Autodesk Inventor part; units mm, degrees
ref_plane "YZ Plane" through (0, 0, 0) normal (1, 0, 0) x (0, 1, 0)
ref_plane "XZ Plane" through (0, 0, 0) normal (0, 1, 0) x (-1, 0, 0)
ref_plane "XY Plane" through (0, 0, 0) normal (0, 0, 1) x (1, 0, 0)
sketch "Esboço4" plane through (0, 0, 0) normal (0, 0, 1) x (1, 0, 0)
  point P0 (0, 0)
  point P1 (43.221, 21.8373)
  point P2 (101.0161, 22.7479)
  point P3 (77.0161, 22.7479)
sketch "Esboço5" plane through (0, 0, 0) normal (0, 0, 1) x (1, 0, 0)
  line L0 (46.357, -8.7268) -> (46.357, 6.1732)
  line L1 (66.357, 6.1732) -> (66.357, -8.7268)
  line L2 (46.357, 6.1732) -> (44.357, 6.1732)
  line L3 (44.357, 6.1732) -> (44.357, -8.7268)
  line L4 (44.357, -8.7268) -> (46.357, -8.7268)
  line L5 (56.357, 6.1732) -> (56.357, -8.7268)
  circle A0 centre (42.407, -1.2768) radius 1.4
  line L6 (39.007, -1.2768) -> (44.357, -6.6268)
  line L7 (39.007, -1.2768) -> (46.573, -1.2768) construction
  line L8 (39.007, -1.2768) -> (39.007, 2.1232)
  line L9 (39.007, 2.1232) -> (44.357, 2.1232)
  line L10 (66.357, -8.7268) -> (66.357, 6.1732)
  line L11 (66.357, 6.1732) -> (68.357, 6.1732)
  line L12 (68.357, 6.1732) -> (68.357, -8.7268)
  line L13 (68.357, -8.7268) -> (66.357, -8.7268)
  circle A1 centre (70.307, -1.2768) radius 1.4
  line L14 (73.707, -1.2768) -> (68.357, -6.6268)
  line L15 (73.707, -1.2768) -> (66.1409, -1.2768) construction
  line L16 (73.707, -1.2768) -> (73.707, 2.1232)
  line L17 (73.707, 2.1232) -> (68.357, 2.1232)
  point P0 (0, 0)
  dimension "d23" = 20
  dimension "d29" = 2
  dimension "d35" = 45
extrude "Extrusão4" add sketch "Esboço5" along normal blind 2
sketch "Esboço6" plane through (0, 0, 2) normal (0, 0, 1) x (1, 0, 0)
  line L0 (46.357, 6.1732) -> (44.357, 6.1732)
  line L1 (46.357, 6.1732) -> (44.357, 6.1732)
  line L2 (44.357, -8.7268) -> (46.357, -8.7268)
  line L3 (46.357, -8.7268) -> (46.357, 6.1732)
  line L4 (44.357, 6.1732) -> (44.357, -8.7268)
  line L5 (46.357, -8.7268) -> (44.357, -8.7268)
  line L6 (66.357, 6.1732) -> (66.357, -8.7268)
  line L7 (68.357, 6.1732) -> (66.357, 6.1732)
  line L8 (66.357, 6.1732) -> (68.357, 6.1732)
  line L9 (68.357, 6.1732) -> (68.357, -8.7268)
  line L10 (68.357, -8.7268) -> (66.357, -8.7268)
  line L11 (66.357, -8.7268) -> (66.357, 6.1732)
  point P0 (0, 0)
extrude "Extrusão5" add sketch "Esboço6" along normal blind 11
sketch "Esboço7" plane through (0, 0, 13) normal (0, 0, 1) x (1, 0, 0)
  line L0 (44.357, 6.1732) -> (44.357, 2.1232)
  line L1 (68.357, -8.7268) -> (68.357, 6.1732)
  line L2 (44.357, 6.1732) -> (68.357, 6.1732)
  line L3 (68.357, 6.1732) -> (68.357, -8.7268)
  line L4 (68.357, -8.7268) -> (44.357, -8.7268)
  line L5 (44.357, -8.7268) -> (44.357, 6.1732)
  point P0 (0, 0)
extrude "Extrusão6" add sketch "Esboço7" along normal blind 2
chamfer "Chanfro1" distance 1 angle 45 1 edges at (68.907, -1.2768, 2)
chamfer "Chanfro2" distance 1 angle 45 1 edges at (41.007, -1.2768, 2)
properties part number "protetor_luz"
Input: part model. Units: mm. Frame: model coordinates. A direction names the side the tool comes from. Give positions to 0.01 mm unless a question says otherwise; leave off trailing zeros. Write each loop counter-clockwise with the first axis right and the second up, starting at its lowest first coordinate (ties: lowest second). Pieces come first, ordered by that corner, then holes. Notation, with made-up numbers: (-1, 7) -> (9, 7) arc R21 cw to (9, 35) -> close; hole circle Ø2 at (52.25, 74.25). An arc over 180 degrees is marked (long way). Use one line per item in the form item = value. Start each with the question number.
1) Pin query (flat end, axial travel): pin 1 (6 mm diameter, centred on y = -4.5, z = 2.5, fed in from -X); pin 2 (1.5 mm diameter, centred on y = -6.5, z = 7, fed in from -X); pin 3 (0.6 mm diameter, centred on x = 42.5, z = 1.5, fed in from +Y). Return the tip coordinate at first contact, or that it passes through.
2) Section query A-A on z = 9. Return the cut outline in (x, y).
3) Set-up query: faces 1 (the flat face through (42, 2.123, 1)), 2 (the flat face through (73, -1, 2)), 3 (the flat face through (71, 2.123, 1)), 4 (the flat face through (46.357, -1, 6)). Return all of +Z, -Z, +X, -X, +Y, -Y with unobstructed straight access to the full face (end or side cutting, diameter ignored); none if empty.
4) Section query D-D on x = 53. Return the cut outline in (y, z), then the cut area to 3 significant figures.
5) Draft query along X for faces 5 (the flat face through (40, 0, 2)), 6 (the flat face through (71.069, -3.914, 0.986)), 7 (the conical face through (71.761, -1.88, 1.174)). Return one class per face: pulls with the +X half, pulls with the -X half, needs draft (parallel to the pull), parting line crosses it, or undercut.
6) Section query B-B on y = 3.25. Return the cut outline in (x, z).
7) Section query C-C on z = 13.5. Return the cut outline in (x, y), then the cut area to 3 significant figures.
8) Ray query, probe 1 along X at (y, z) = (-4.25, 11); probe 2 along Z at (x, y) = (59, -5.5); probe 3 along X at (y, z) = (-5.5, 1.75). Return the intervals inside material, ascending. Write a range as from..to.
Outcome:
q1.pin_1 = 39.27
q1.pin_2 = 44.36
q1.pin_3 = 2.12
q2.outline = (44.36, -8.73) -> (46.36, -8.73) -> (46.36, 6.17) -> (44.36, 6.17) -> close; (66.36, -8.73) -> (68.36, -8.73) -> (68.36, 6.17) -> (66.36, 6.17) -> close
q3.face_1 = +Z, -Z, -X, +Y
q3.face_2 = +Z, +X, +Y, -Y
q3.face_3 = +Z, -Z, +X, +Y
q3.face_4 = -Z, +Y, -Y
q4.outline = (-8.73, 13) -> (6.17, 13) -> (6.17, 15) -> (-8.73, 15) -> close
q4.area = 29.8 mm^2
q5.face_5 = needs draft
q5.face_6 = pulls with the +X half
q5.face_7 = undercut
q6.outline = (44.36, 0) -> (46.36, 0) -> (46.36, 13) -> (66.36, 13) -> (66.36, 0) -> (68.36, 0) -> (68.36, 15) -> (44.36, 15) -> close
q7.outline = (44.36, -8.73) -> (68.36, -8.73) -> (68.36, 6.17) -> (44.36, 6.17) -> close
q7.area = 358 mm^2
q8.probe_1 = 44.36..46.36, 66.36..68.36
q8.probe_2 = 13..15
q8.probe_3 = 43.23..46.36, 66.36..69.48
